Geometry: see drawing. Coordinates: mm, zero at the bounding-box minimum. A direction names the side the tool comes from. Give positions to 0.01 mm unless a question says otherwise; leave off trailing zeros. Loops run counter-clockwise (first coordinate to the right, second up) from the corner with the lowest first, then second, coordinate; pieces in that order, holes last. Notation, with made-up numbers: (64.25, 35.5) - (111.25, 35.5) arc R24 cw to (111.25, 53.5) - close; hole circle Ø10 at (52.5, 58.25). An arc over 180 degrees is marked (long way). Use one line per item in the form item = value.
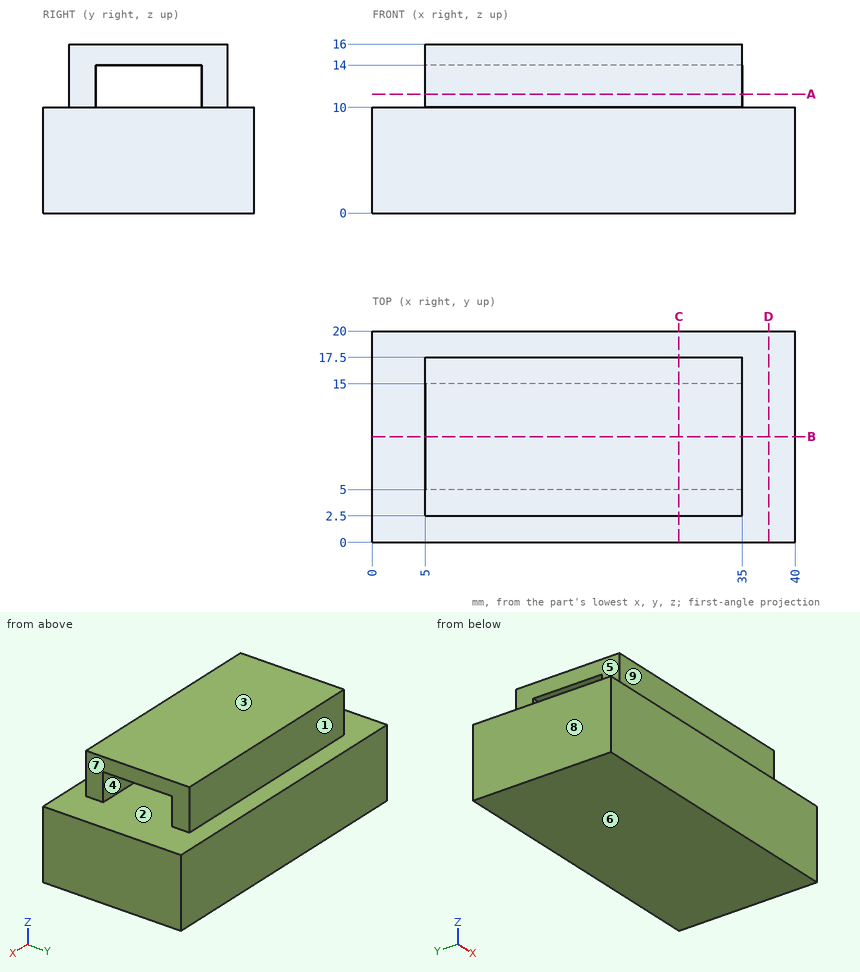
(1) Cut plane A-A (z = 11.25). Return the cut outline in (x, y).
Solution:
outline = (5, 2.5) - (35, 2.5) - (35, 5) - (5, 5) - close; (5, 15) - (35, 15) - (35, 17.5) - (5, 17.5) - close
(2) Access query for the marked faces 5, 6, 7, 8 and 9. Directions: +Z, -Z, +X, -X, +Y, -Y. A direction counts if a zero-diameter tool reaches every point of the face in a straight line with its end or side. Return the directions, or none.
Solution:
face_5 = +Z, -X, +Y, -Y
face_6 = -Z, +X, -X, +Y, -Y
face_7 = +Z, +X, +Y, -Y
face_8 = +Z, -Z, -X, +Y, -Y
face_9 = +Z, +X, -X, -Y
(3) Cut plane D-D (x = 37.5). Return the cut outline in (y, z).
Solution:
outline = (0, 0) - (20, 0) - (20, 10) - (0, 10) - close
(4) Cut plane C-C (x = 29). Return the cut outline in (y, z).
Solution:
outline = (0, 0) - (20, 0) - (20, 10) - (17.5, 10) - (17.5, 16) - (2.5, 16) - (2.5, 10) - (0, 10) - close; hole (5, 10) - (15, 10) - (15, 14) - (5, 14) - close
(5) Cut plane B-B (y = 10). Return the cut outline in (x, z).
Solution:
outline = (0, 0) - (40, 0) - (40, 10) - (0, 10) - close; (5, 14) - (35, 14) - (35, 16) - (5, 16) - close
(6) Pull-direction query (Y, two-part tool) for the marked faces 1, 2, 3 and 4; classes: released by +Y, released by -Y, zero draft, split by the parting line, or undercut.
Solution:
face_1 = released by +Y
face_2 = undercut
face_3 = zero draft
face_4 = undercut
(7) Material intervals for L1, parallel to Y at x = 15, z = 12.75; L2, parallel to Z at x = 18, y = 12.25; L3, parallel to Z at x = 15, y = 1.25, sorted ascending. Write a range as from..to.
Solution:
L1 = 2.5..5, 15..17.5
L2 = 0..10, 14..16
L3 = 0..10
(8) Pin query (flat end, axial travel): P1, Ø1.2, axis at x = 21, z = 12, coming from the -Y side; P2, Ø1.8, axis at y = 8, z = 12, coming from the -X side; P3, Ø3, axis at x = 17.5, z = 13, coming from the +Y side; P4, Ø1.5, axis at y = 2.5, z = 12.5, coming from the -X side. Return the tip coordinate at first contact, or that it passes through.
Solution:
P1 = 2.5
P2 = through
P3 = 17.5
P4 = 5
